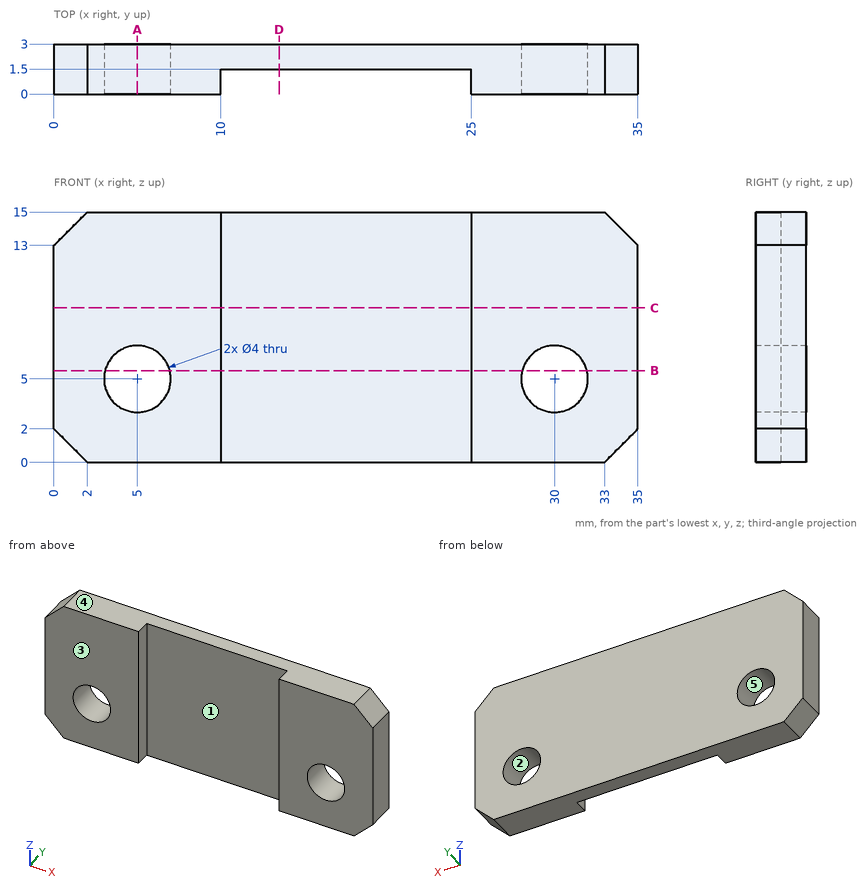
Check sheet for the drawn part. Datum: minimum x, y, z corner. Units: mm. A direction names the side the tool comes from. Coordinates: 2 decimals unless noted, no trailing zeros. Order: outer loops, then holes, each group sorted by start corner. A loop starts at its lowest first (then second) coordinate and runs counter-clockwise, first axis right, second up. Notation, with made-up numbers: M -28.5,3.25 L -5.5,3.25 A10 cw -5.5,17.25 Z; hole C 21.25,2.25 d11. An arc over 180 degrees is marked long. One line per question, with ' | ' between items. Start each with the question number.
Item 1: Mould release check, pull along Z, two halves, no side actions. Record for the marked faces 3, 4 and 5: pulls with the +Z half, pulls with the -Z half, needs draft (parallel to the pull), parting line crosses it, or undercut.
Item 2: Gauge pin test, flat ends, axial feed: P1, Ø1.6, axis at y = 1, z = 8.5, coming from the -X side; P2, Ø1, axis at x = 21, z = 6, coming from the -Y side. Record the tip position at first contact, or that the pin passes through.
Item 3: Sectioned sample at B-B on z = 5.5. Record the cut outline in (x, y), and give its area (3 significant figures).
Item 4: Sectioned sample at D-D on x = 13.5. Record the cut outline in (y, z), and give its area (3 significant figures).
Item 5: Sectioned sample at C-C on z = 9.25. Record the cut outline in (x, y).
Item 6: Access from +Z, -Z, +X, -X, +Y, -Y to the whole of each face (thin tool, end or side, straight path). Record for the marked faces 1 and 2.
Item 7: Material ranges on line 1 (X direction, y = 0.9, z = 11.5); line 2 (Z direction, x = 30, y = 1.75); line 3 (Y direction, x = 15.5, z = 10.5), recorded low to high.
Item 8: Sectioned sample at A-A on x = 5. Record the cut outline in (y, z).
Answer below:
1) face 3: needs draft | face 4: pulls with the +Z half | face 5: undercut
2) P1: stops at x = 0 | P2: stops at y = 1.5
3) outline: M 0,0 L 3.06,0 L 3.06,3 L 0,3 Z; M 6.94,0 L 10,0 L 10,1.5 L 25,1.5 L 25,0 L 28.06,0 L 28.06,3 L 6.94,3 Z; M 31.94,0 L 35,0 L 35,3 L 31.94,3 Z | area: 59.3 mm^2
4) outline: M 1.5,0 L 3,0 L 3,15 L 1.5,15 Z | area: 22.5 mm^2
5) outline: M 0,0 L 10,0 L 10,1.5 L 25,1.5 L 25,0 L 35,0 L 35,3 L 0,3 Z
6) face 1: +Z, -Z, -Y | face 2: +Y, -Y
7) line 1: x = 0 to 10, 25 to 35 | line 2: z = 0 to 3, 7 to 15 | line 3: y = 1.5 to 3
8) outline: M 0,0 L 3,0 L 3,3 L 0,3 Z; M 0,7 L 3,7 L 3,15 L 0,15 Z
